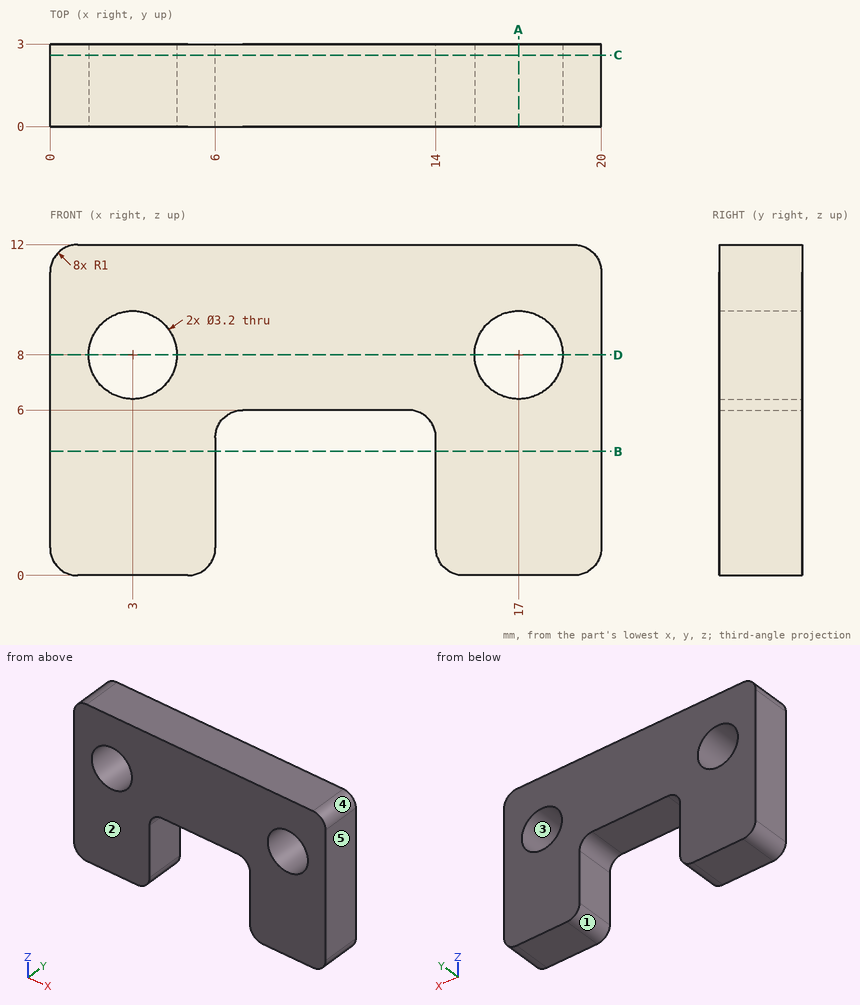
For this review, use the dimensioned drawing (mm, ordinates from the lowest corner) and the shaded views. A direction names the side the tool comes from. Give positions to 0.01 mm unless a question says otherwise; leave off trailing zeros. Order: outer loops, then holes, each group sorted by start corner. A loop starts at its lowest first (then second) coordinate and runs counter-clockwise, first axis right, second up. Notation, with made-up numbers: (-0.75, 37) - (49.25, 37) arc R15 ccw to (49.25, 49) - close; hole circle Ø4 at (28.25, 59.5). An arc over 180 degrees is marked (long way). Use a Markdown table: item, result. Add a question column.
(1) Wall thickness on probe 1 along X at (y, z) = (1.6, 8); probe 2 along Z at (x, y) = (3, 1.9); probe 3 along X at (y, z) = (1.15, 7): over which ranges is each line inside the solid? List them lowest first. Write a range as [from, to].
(2) Add section D-D on z = 8. Give the boundary of the cut face in (x, y), then the cut area to 3 significant figures.
(3) Add section C-C on y = 2.6. Give the boundary of the cut face in (x, z).
(4) Add section A-A on x = 17. Give the boundary of the cut face in (y, z), then the cut area to 3 significant figures.
(5) Clearance check with flat-ended pins moving along their axes: P1, Ø1.5, axis at x = 9, y = 1, coming from the -Z side; P2, Ø4, axis at x = 17, z = 8, coming from the +Y side; P3, Ø2.5, axis at x = 3, z = 8, coming from the +Y side. State where each tip first meets the part, or that it passes through.
(6) Machinability: for the marked faces 1 and 2, which of the approach directions +Z, -Z, +X, -X, +Y, -Y give a long, thin tool a straight path to every point of the face, cutting with its end or side? Answer none if there is none.
(7) Add section B-B on z = 4.5. Give the boundary of the cut face in (x, y), then the cut area to 3 significant figures.
(8) Mouldability with a two-part tool opening along Z and no side actions: class the marked faces 3, 4 and 5 as +Z half, -Z half, draft (parallel to the pull), parting line (faces both ways), or undercut.
Report:
| question | item | result |
|---|---|---|
| 1 | probe 1 | x = [0, 1.4], [4.6, 15.4], [18.6, 20] |
| 1 | probe 2 | z = [0, 6.4], [9.6, 12] |
| 1 | probe 3 | x = [0, 1.75], [4.25, 15.75], [18.25, 20] |
| 2 | outline | (0, 0) - (1.4, 0) - (1.4, 3) - (0, 3) - close; (4.6, 0) - (15.4, 0) - (15.4, 3) - (4.6, 3) - close; (18.6, 0) - (20, 0) - (20, 3) - (18.6, 3) - close |
| 2 | area | 40.8 mm² |
| 3 | outline | (0, 1) arc R1 ccw to (1, 0) - (5, 0) arc R1 ccw to (6, 1) - (6, 5) arc R1 cw to (7, 6) - (13, 6) arc R1 cw to (14, 5) - (14, 1) arc R1 ccw to (15, 0) - (19, 0) arc R1 ccw to (20, 1) - (20, 11) arc R1 ccw to (19, 12) - (1, 12) arc R1 ccw to (0, 11) - close; hole circle Ø3.2 at (3, 8); hole circle Ø3.2 at (17, 8) |
| 4 | outline | (0, 0) - (3, 0) - (3, 6.4) - (0, 6.4) - close; (0, 9.6) - (3, 9.6) - (3, 12) - (0, 12) - close |
| 4 | area | 26.4 mm² |
| 5 | P1 | stops at z = 6 |
| 5 | P2 | stops at y = 3 |
| 5 | P3 | passes through |
| 6 | face 1 | -Z, +Y, -Y |
| 6 | face 2 | +Z, -Z, +X, -X, -Y |
| 7 | outline | (0, 0) - (6, 0) - (6, 3) - (0, 3) - close; (14, 0) - (20, 0) - (20, 3) - (14, 3) - close |
| 7 | area | 36.0 mm² |
| 8 | face 3 | undercut |
| 8 | face 4 | +Z half |
| 8 | face 5 | draft |
